Part model, mm, in its own coordinate system. Face numbers are marked on the shaded views. A direction names the side the tool comes from. Give positions to 0.01 mm unless a question says otherwise; leave off trailing zeros. Order: outer loops, then holes, each group sorted by start corner. A loop starts at its lowest first (then second) coordinate and runs counter-clockwise, first axis right, second up. Notation, with made-up numbers: (42.5, 78.5) - (92.5, 78.5) arc R21 cw to (92.5, 83.5) - close; hole circle Ø6 at (70, 17). An arc over 180 degrees is marked (long way). One line per item, written item: value.
```python
from build123d import *

# Parameters (mm, degrees)
F2_SIZE = 0.5


with BuildPart() as f1:
    # F0 (on Top) → F1 (revolve)
    with BuildSketch(Plane.XY):
        Polygon((-51.3, 11.5), (-51.3, 10.2), (0, 10.2), (0, 15.75), (-2.3, 15.75), (-2.3, 13), (-13.5, 13), (-13.5, 15.75), (-15.8, 15.75), (-15.8, 11.5), align=None)
    revolve(axis=Axis((-27.94127, 0, 0), (-1, 0, 0)))

    # F2
    f2_edges = [f1.edges().sort_by_distance(p)[0] for p in [
        (-51.3, -11.5, 0),
        (0, -10.2, 0),
    ]]
    chamfer(f2_edges, length=F2_SIZE)


solid = f1.part
```
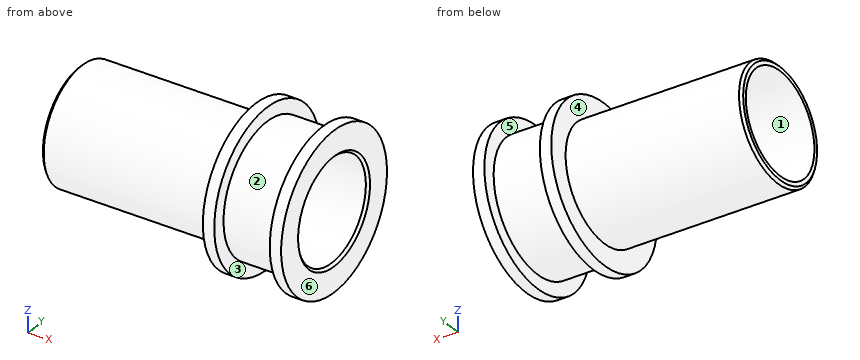
1) Drill centre lines: line 1 along Z through (x, y) = (-31, 0); line 2 along X through (y, z) = (-14, -1). Where is each one in solid material? Low to high. Write a range as from..to.
Outcome:
line 1: z = -11.5..-10.2, 10.2..11.5
line 2: x = -15.8..-13.5, -2.3..0
2) Cut at A-A, the plane y = 0. Give the cut face in (x, z).
Outcome:
outline: (-51.3, -11) - (-50.8, -11.5) - (-15.8, -11.5) - (-15.8, -15.75) - (-13.5, -15.75) - (-13.5, -13) - (-2.3, -13) - (-2.3, -15.75) - (0, -15.75) - (0, -10.7) - (-0.5, -10.2) - (-51.3, -10.2) - close; (-51.3, 10.2) - (-0.5, 10.2) - (0, 10.7) - (0, 15.75) - (-2.3, 15.75) - (-2.3, 13) - (-13.5, 13) - (-13.5, 15.75) - (-15.8, 15.75) - (-15.8, 11.5) - (-50.8, 11.5) - (-51.3, 11) - close
3) Pin check, flat tips, straight feed: pin 1 (1.5 mm diameter, centred on y = 10, z = -11.5, fed in from -X); pin 2 (4 mm diameter, centred on x = -6.5, y = 0.5, fed in from +Z); pin 3 (1.5 mm diameter, centred on x = -11, z = -5, fed in from -Y). Stop position of each tip, or through.
Outcome:
pin 1: stops at x = -15.8
pin 2: stops at z = 13
pin 3: stops at y = -12.29
4) Which spindle directions (+Z, -Z, +X, -X, +Y, -Y) get a long thin tool onto all of the face, cutting with end or side? Do the marked faces 4, 5 and 6. Say none if no direction does.
Outcome:
face 4: -X
face 5: none
face 6: +Z, -Z, +X, +Y, -Y
5) Cut at D-D, the plane x = -6. Give the cut face in (y, z), then the cut area to 3 significant figures.
Outcome:
outline: circle Ø26 at (0, 0); hole circle Ø20.4 at (0, 0)
area: 204 mm^2
6) Mould opens along Z. For the marked faces 1, 2 and 3 say: released by +Z, released by -Z, zero draft, split by the parting line, or undercut.
Outcome:
face 1: undercut
face 2: split by the parting line
face 3: zero draft
7) Cut at C-C, the plane x = -25.5. Give the cut face in (y, z), then the cut area to 3 significant figures.
Outcome:
outline: circle Ø23 at (0, 0); hole circle Ø20.4 at (0, 0)
area: 88.6 mm^2
